Verification items for the finished model (mm, model axes). A direction names the side the tool comes from. Round coordinates to 2 decimals unless told otherwise and drop trailing zeros. Write each loop counter-clockwise with the first axis right and the second up, starting at its lowest first coordinate (ties: lowest second). Pieces come first, ordered by that corner, then holes. Notation, with made-up numbers: (46.5, 14) -> (62.5, 14) arc R14 cw to (62.5, 21) -> close; hole circle Ø2 at (37, 85). An arc over 180 degrees is marked (long way). Use CSV: the item, a comma, the result in double quotes.
```python
from build123d import *

# Parameters (mm, degrees)
SKETCH1_W           = 600
SKETCH1_H           = 600
SKETCH1_R           = 3
SKETCH1_R_2         = 1.5
BOSS_EXTRUDE1_DEPTH = 12


with BuildPart() as part:
    # Sketch1 → Boss-Extrude1 (new body)
    with BuildSketch(Plane(origin=(0, 0, 0), x_dir=(1, 0, 0), z_dir=(0, 1, 0))):
        Rectangle(SKETCH1_W, SKETCH1_H)
        with Locations(Location((0, 250, 0), (0, 0, 270))):
            Circle(SKETCH1_R, mode=Mode.SUBTRACT)
        with Locations(Location((77.254248594, 237.764129074, 0), (0, 0, 270))):
            Circle(SKETCH1_R, mode=Mode.SUBTRACT)
        with Locations(Location((146.946313073, 202.254248594, 0), (0, 0, 270))):
            Circle(SKETCH1_R, mode=Mode.SUBTRACT)
        with Locations(Location((202.254248594, 146.946313073, 0), (0, 0, 270))):
            Circle(SKETCH1_R, mode=Mode.SUBTRACT)
        with Locations(Location((237.764129074, 77.254248594, 0), (0, 0, 270))):
            Circle(SKETCH1_R, mode=Mode.SUBTRACT)
        with Locations(Location((250, 0, 0), (0, 0, 270))):
            Circle(SKETCH1_R, mode=Mode.SUBTRACT)
        with Locations(Location((237.764129074, -77.254248594, 0), (0, 0, 270))):
            Circle(SKETCH1_R, mode=Mode.SUBTRACT)
        with Locations(Location((202.254248594, -146.946313073, 0), (0, 0, 270))):
            Circle(SKETCH1_R, mode=Mode.SUBTRACT)
        with Locations(Location((146.946313073, -202.254248594, 0), (0, 0, 270))):
            Circle(SKETCH1_R, mode=Mode.SUBTRACT)
        with Locations(Location((77.254248594, -237.764129074, 0), (0, 0, 270))):
            Circle(SKETCH1_R, mode=Mode.SUBTRACT)
        with Locations(Location((0, -250, 0), (0, 0, 270))):
            Circle(SKETCH1_R, mode=Mode.SUBTRACT)
        with Locations(Location((-77.254248594, -237.764129074, 0), (0, 0, 270))):
            Circle(SKETCH1_R, mode=Mode.SUBTRACT)
        with Locations(Location((-146.946313073, -202.254248594, 0), (0, 0, 270))):
            Circle(SKETCH1_R, mode=Mode.SUBTRACT)
        with Locations(Location((-202.254248594, -146.946313073, 0), (0, 0, 270))):
            Circle(SKETCH1_R, mode=Mode.SUBTRACT)
        with Locations(Location((-237.764129074, -77.254248594, 0), (0, 0, 270))):
            Circle(SKETCH1_R, mode=Mode.SUBTRACT)
        with Locations(Location((-250, 0, 0), (0, 0, 270))):
            Circle(SKETCH1_R, mode=Mode.SUBTRACT)
        with Locations(Location((-237.764129074, 77.254248594, 0), (0, 0, 270))):
            Circle(SKETCH1_R, mode=Mode.SUBTRACT)
        with Locations(Location((-202.254248594, 146.946313073, 0), (0, 0, 270))):
            Circle(SKETCH1_R, mode=Mode.SUBTRACT)
        with Locations(Location((-146.946313073, 202.254248594, 0), (0, 0, 270))):
            Circle(SKETCH1_R, mode=Mode.SUBTRACT)
        with Locations(Location((-77.254248594, 237.764129074, 0), (0, 0, 270))):
            Circle(SKETCH1_R, mode=Mode.SUBTRACT)
        with Locations(Location((-250, 250, 0), (0, 0, 270))):
            Circle(SKETCH1_R_2, mode=Mode.SUBTRACT)
        with Locations(Location((250, 250, 0), (0, 0, 270))):
            Circle(SKETCH1_R_2, mode=Mode.SUBTRACT)
        with Locations(Location((250, -250, 0), (0, 0, 270))):
            Circle(SKETCH1_R_2, mode=Mode.SUBTRACT)
        with Locations(Location((-250, -250, 0), (0, 0, 270))):
            Circle(SKETCH1_R_2, mode=Mode.SUBTRACT)
        with BuildLine():
            Line((-203.190468868, 99.063784307), (-199.902587408, -6.241437954))
            ThreePointArc((-199.902587408, -6.241437954), (-173.205080757, -100), (-105.356537529, -170))
            Line((-105.356537529, -170), (-15.803480629, -225.5))
            ThreePointArc((-15.803480629, -225.5), (0, -230), (15.803480629, -225.5))
            Line((15.803480629, -225.5), (105.356537529, -170))
            ThreePointArc((105.356537529, -170), (173.205080757, -100), (199.902587408, -6.241437954))
            Line((199.902587408, -6.241437954), (203.190468868, 99.063784307))
            ThreePointArc((203.190468868, 99.063784307), (199.18584287, 115), (187.386988239, 126.436215693))
            Line((187.386988239, 126.436215693), (94.546049879, 176.241437954))
            ThreePointArc((94.546049879, 176.241437954), (0, 200), (-94.546049879, 176.241437954))
            Line((-94.546049879, 176.241437954), (-187.386988239, 126.436215693))
            ThreePointArc((-187.386988239, 126.436215693), (-199.18584287, 115), (-203.190468868, 99.063784307))
        make_face(mode=Mode.SUBTRACT)
    extrude(amount=BOSS_EXTRUDE1_DEPTH)


solid = part.part
```
Q1. Section check B-B (x = -114.5). Record the cut outline in (y, z), plus the area to 3 significant figures.
Filled in:
outline,"(0, -300) -> (12, -300) -> (12, -165.54) -> (0, -165.54) -> close; (0, 163.98) -> (12, 163.98) -> (12, 300) -> (0, 300) -> close"
area,"3,250 mm²"
Q2. Access from +Z, -Z, +X, -X, +Y, -Y to the whole of each face (thin tool, end or side, straight path). Record for faces 1 (the flat face through (-204, 0, -4)), 2 (the cylindrical face through (199.3, 5.9, -114.8)).
Filled in:
face 1,"+Z, -Z, +X, -X, -Y"
face 2,"+Y, -Y"
Q3. Material ranges on L1, parallel to X at y = 4.75, z = -250; L2, parallel to X at y = 11.5, z = 15; L3, parallel to X at y = 2.75, z = 183, recorded low to high.
Filled in:
L1,"-300 to -251.5, -248.5 to -3, 3 to 248.5, 251.5 to 300"
L2,"-300 to -199.44, 199.44 to 300"
L3,"-300 to -84.38, 84.38 to 300"
Q4. Go/stop test with a flat-tipped pin: P1, Ø5.5, axis at x = 77.25, z = 237.76, coming from the -Y side (3 decimals). Record where the tip stops, or that it passes through.
Filled in:
P1,"through"
Q5. Section check A-A (z = 92). Record the cut outline in (x, y).
Filled in:
outline,"(-300, 0) -> (-177.58, 0) -> (-177.58, 12) -> (-300, 12) -> close; (177.58, 0) -> (300, 0) -> (300, 12) -> (177.58, 12) -> close"
Q6. Mould release check, pull along Z, two halves, no side actions. Record for faces 3 (the flat face through (59.95, 5.92, 198.14)), 4 (the flat face through (-204, 12, -4)): released by +Z, released by -Z, zero draft, split by the parting line, or undercut.
Filled in:
face 3,"undercut"
face 4,"zero draft"
Q7. Section check C-C (y = 5.25). State how many separate pieces and enclosed holes the cut face has, plus the area to 3 significant figures.
Filled in:
separate pieces,"1"
enclosed holes,"25"
area,"226,000 mm²"
